Geometry check sheet. Reference: the model listing, model coordinates, mm. Face numbers are marked on the shaded views. Coordinates: 2 decimals unless noted, no trailing zeros. Write each loop counter-clockwise with the first axis right and the second up, starting at its lowest first coordinate (ties: lowest second). Pieces come first, ordered by that corner, then holes. Notation, with made-up numbers: (-4.75, -19.5) -> (28.25, -19.5) arc R27 ccw to (28.25, 1.5) -> close; hole circle Ø1 at (20.5, -17.5). An arc over 180 degrees is marked (long way). One line per question, with ' | ' between items.
from build123d import *

# Parameters (mm, degrees)
F0_W     = 21
F0_H     = 82
F1_DEPTH = 2
F3_DEPTH = 2
F6_DEPTH = 2


with BuildPart() as f1:
    # F0 (on Top) → F1 (new body)
    with BuildSketch(Plane.XY):
        with Locations((-21.0416306257, 2.1058048904)):
            Rectangle(F0_W, F0_H)
    extrude(amount=F1_DEPTH)

    # F2 (on face) → F3 (join)
    with BuildSketch(Plane.XY.offset(2)):
        Polygon((-12.5416306257, -38.8941951096), (-10.5416306257, -38.8941951096), (-10.5416306257, 43.1058048904), (-31.5416306257, 43.1058048904), (-31.5416306257, -38.8941951096), (-29.5416306257, -38.8941951096), (-29.5416306257, 41.1058048904), (-12.5416306257, 41.1058048904), align=None)
    extrude(amount=F3_DEPTH)

    # F5 (on offset) → F6 (join)
    with BuildSketch(Plane.XY.offset(4)):
        Polygon((-10.5416306257, 8.1058048904), (-10.5416306257, 43.1058048904), (-31.5416306257, 43.1058048904), (-31.5416306257, 8.1058048904), (-31.5416306257, 0), (-31.5416306257, -38.8941951096), (-27.5416306257, -38.8941951096), (-27.5416306257, 6.1058048904), (-14.5416306257, 6.1058048904), (-14.5416306257, -38.8941951096), (-10.5416306257, -38.8941951096), align=None)
    extrude(amount=F6_DEPTH)


solid = f1.part
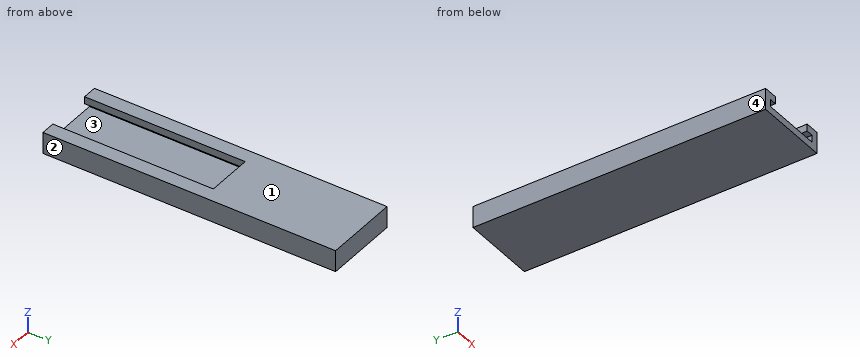
1. Cross-section at A-A on z = 5. Record the boundary of the cut face in (x, y).
Worked answers:
outline: (-31.54, -38.89) -> (-27.54, -38.89) -> (-27.54, 6.11) -> (-14.54, 6.11) -> (-14.54, -38.89) -> (-10.54, -38.89) -> (-10.54, 43.11) -> (-31.54, 43.11) -> close
2. Material ranges on line 1 (Z direction, x = -28, y = 30); line 2 (X direction, y = -23, z = 4.7); line 3 (X direction, y = 35.5, z = 3.1), recorded low to high. Write a range as from..to.
Worked answers:
line 1: 0..2, 4..6 | line 2: -31.54..-27.54, -14.54..-10.54 | line 3: -31.54..-29.54, -12.54..-10.54
3. Cross-section at D-D on y = -17.5. Record the boundary of the cut face in (x, z).
Worked answers:
outline: (-31.54, 0) -> (-10.54, 0) -> (-10.54, 6) -> (-14.54, 6) -> (-14.54, 4) -> (-12.54, 4) -> (-12.54, 2) -> (-29.54, 2) -> (-29.54, 4) -> (-27.54, 4) -> (-27.54, 6) -> (-31.54, 6) -> close
4. Go/stop test with flat-tipped pins: P1, Ø1, axis at x = -20, z = 3, coming from the -Y side; P2, Ø1, axis at x = -21.5, z = 5, coming from the -Y side; P3, Ø12, axis at x = -20, y = -4, coming from the -Z side. Record where each tip stops, or that it passes through.
Worked answers:
P1: y = 41.11 | P2: y = 6.11 | P3: z = 0
5. Cross-section at C-C on x = -23.25. Record the boundary of the cut face in (y, z), and give its area (3 significant figures).
Worked answers:
outline: (-38.89, 0) -> (43.11, 0) -> (43.11, 6) -> (6.11, 6) -> (6.11, 4) -> (41.11, 4) -> (41.11, 2) -> (-38.89, 2) -> close | area: 242 mm²
6. Mould release check, pull along X, two halves, no side actions. Record for the marked faces 1, 2, 3 and 4: released by +X, released by -X, zero draft, split by the parting line, or undercut.
Worked answers:
face 1: zero draft | face 2: released by +X | face 3: undercut | face 4: released by -X
7. Cross-section at B-B on y = 20.5. Record the boundary of the cut face in (x, z), and give its area (3 significant figures).
Worked answers:
outline: (-31.54, 0) -> (-10.54, 0) -> (-10.54, 6) -> (-31.54, 6) -> close; hole (-29.54, 2) -> (-12.54, 2) -> (-12.54, 4) -> (-29.54, 4) -> close | area: 92.0 mm²
